The drawing under review shows one solid part. Ordinate dimensions are in mm from its lowest x, y, z. Round coordinates to 2 decimals unless told otherwise and drop trailing zeros. Order: outer loops, then holes, each group sorted by start corner. A loop starts at its lowest first (then second) coordinate and runs counter-clockwise, first axis right, second up. Notation, with made-up numbers: M -16,49.25 L 28,49.25 A6 cw 28,55.25 Z; hole C -19.5,-7.75 d8. An arc over 180 degrees is marked long. Answer as a JSON object with one key per item and string values. Group by question number.
1) Insertion check: pin 1 Ø5.5 at (y, z) = (96.5, 96.5) entering from +X. The pin has a flat end and moves straight along its axis. Give the tip position at first contact, or say it passes through.
2) To check wall thickness, follow line 1 (Z direction, x = 1, y = 96.5); line 2 (Z direction, x = 0.35, y = 95.5). State the ranges of each line that lie inside material, in increasing order.
3) Consider section A-A, the plane z = 96.5. Write out the cut boundary in (x, y).
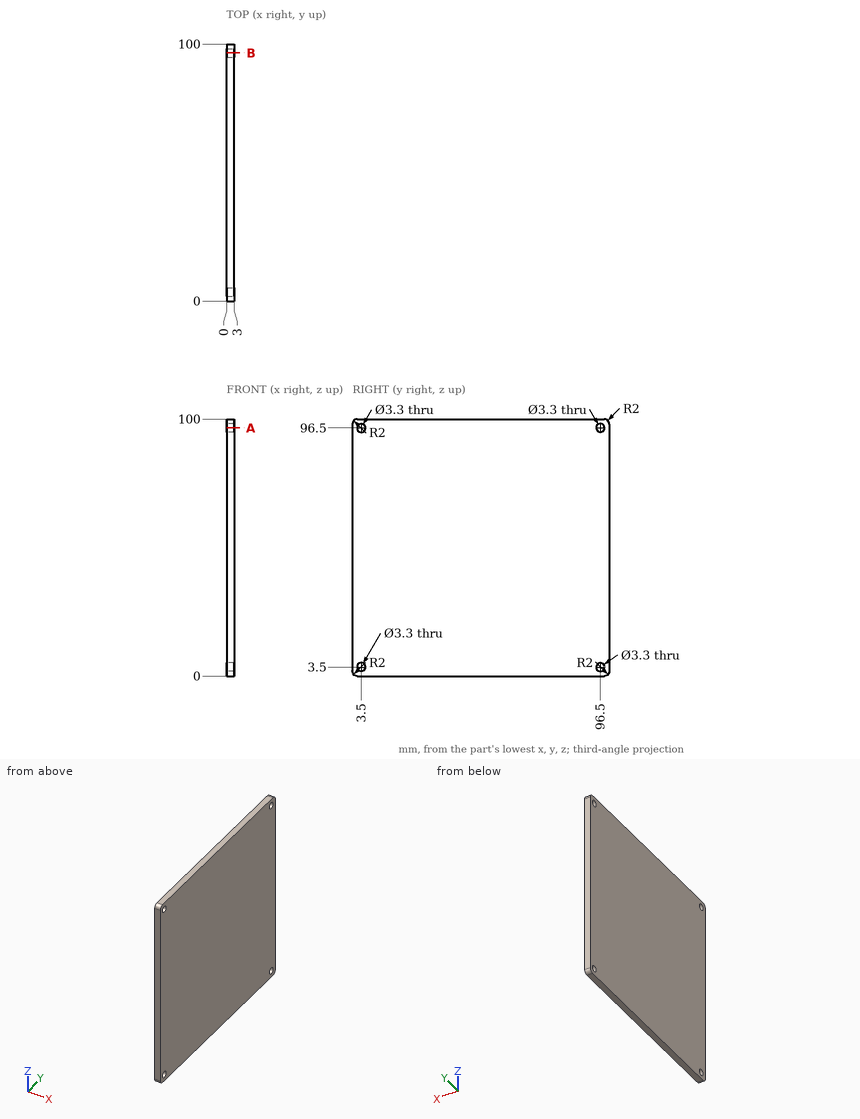
Results list:
{
 "1": {"pin 1": "x = 3"},
 "2": {"line 1": "0 to 1.85, 5.15 to 94.85, 98.15 to 100", "line 2": "0 to 2.19, 4.81 to 95.19, 97.81 to 100"},
 "3": {"outline": "M 0,0 L 3,0 L 3,1.85 L 0,1.85 Z; M 0,5.15 L 3,5.15 L 3,94.85 L 0,94.85 Z; M 0,98.15 L 3,98.15 L 3,100 L 0,100 Z"}
}
